Build history of the part. All positions in model axes, mm. Round coordinates to 2 decimals unless told otherwise and drop trailing zeros. Loops run counter-clockwise (first coordinate to the right, second up) from the corner with the lowest first, then second, coordinate; pieces in that order, holes last. Notation, with made-up numbers: (82.25, -1.5) -> (122.25, -1.5) arc R14 cw to (122.25, 19.5) -> close; hole circle Ø3 at (60, 11.25). An arc over 180 degrees is marked (long way). Put each result on its own line as item: value. Start each with the question number.
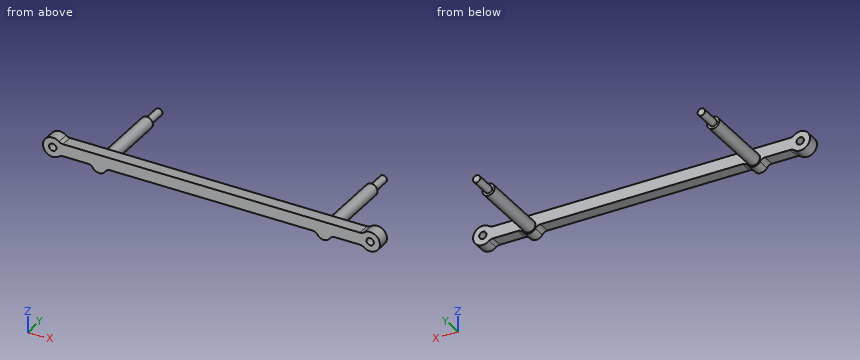
```python
from build123d import *

# Parameters (mm, degrees)
SKETCH1_R           = 1.5
BOSS_EXTRUDE1_DEPTH = 5
FILLET1_R           = 2.5
SKETCH2_R           = 2.5
BOSS_EXTRUDE2_DEPTH = 29
SKETCH3_R           = 1.5
BOSS_EXTRUDE3_DEPTH = 8.5


with BuildPart() as part:
    # Sketch1 → Boss-Extrude1 (new body)
    with BuildSketch(Plane(origin=(0, 0, 0), x_dir=(1, 0, 0), z_dir=(0, 1, 0))):
        with BuildLine():
            Line((-48.958039892, 2.5), (-61.877501001, 2.5))
            ThreePointArc((-61.877501001, 2.5), (-69, 0), (-61.877501001, -2.5))
            Line((-61.877501001, -2.5), (61.877501001, -2.5))
            ThreePointArc((61.877501001, -2.5), (69, 0), (61.877501001, 2.5))
            Line((61.877501001, 2.5), (48.958039892, 2.5))
            ThreePointArc((48.958039892, 2.5), (46, 5), (43.041960108, 2.5))
            Line((43.041960108, 2.5), (-43.041960108, 2.5))
            ThreePointArc((-43.041960108, 2.5), (-46, 5), (-48.958039892, 2.5))
        make_face()
        with Locations((-65, 0)):
            Circle(SKETCH1_R, mode=Mode.SUBTRACT)
        with Locations((65, 0)):
            Circle(SKETCH1_R, mode=Mode.SUBTRACT)
    extrude(amount=BOSS_EXTRUDE1_DEPTH)

    # Fillet1
    fillet1_edges = [part.edges().sort_by_distance(p)[0] for p in [
        (61.877501001, 2.5, -2.5),
        (61.877501001, 2.5, 2.5),
        (-61.877501001, 2.5, 2.5),
        (-61.877501001, 2.5, -2.5),
        (-48.958039892, 2.5, -2.5),
        (-43.041960108, 2.5, -2.5),
        (43.041960108, 2.5, -2.5),
        (48.958039892, 2.5, -2.5),
    ]]
    fillet(fillet1_edges, radius=FILLET1_R)

    # Sketch2 → Boss-Extrude2 (add)
    with BuildSketch(Plane(origin=(0, 5, 0), x_dir=(1, 0, 0), z_dir=(0, 1, 0))):
        with Locations((-46, 2)):
            Circle(SKETCH2_R)
        with Locations((46, 2)):
            Circle(SKETCH2_R)
    extrude(amount=BOSS_EXTRUDE2_DEPTH)

    # Sketch3 → Boss-Extrude3 (add)
    with BuildSketch(Plane(origin=(0, 34, 0), x_dir=(1, 0, 0), z_dir=(0, 1, 0))):
        with Locations((-46, 2)):
            Circle(SKETCH3_R)
        with Locations((46, 2)):
            Circle(SKETCH3_R)
    extrude(amount=BOSS_EXTRUDE3_DEPTH)


solid = part.part
```
Item 1: Cut at A-A on x = -65. Write the cut outline in (y, z), then the cut area to 3 significant figures.
Item 2: Cut at B-B on y = 13. Write the cut outline in (x, z).
Item 3: Cut at D-D on x = 37.5. Write the cut outline in (y, z), then the cut area to 3 significant figures.
Item 4: Drop flat-ended pins along their axis: pin 1 (5.5 mm diameter, centred on x = 14, y = 2.5, fed in from +Z); pin 2 (4 mm diameter, centred on x = -54, y = 2.5, fed in from -Z); pin 3 (4.5 mm diameter, centred on x = -10.5, z = -1.5, fed in from +Y). Give the stop position or say it passes through.
Item 5: Wall check: line 1 (X direction, y = 2.1, z = 0); line 2 (X direction, y = 9.5, z = -2); line 3 (Z direction, x = 65, y = 3). Give the ranges that are in metal, low to high. Write a range as from..to.
Item 6: Cut at C-C on x = -46. Write the cut outline in (y, z), then the cut area to 3 significant figures.
Ans:
1. outline: (0, -4) -> (5, -4) -> (5, -1.5) -> (0, -1.5) -> close; (0, 1.5) -> (5, 1.5) -> (5, 4) -> (0, 4) -> close
1. area: 25.0 mm2
2. outline: circle Ø5 at (-46, -2); circle Ø5 at (46, -2)
3. outline: (0, -2.5) -> (5, -2.5) -> (5, 2.5) -> (0, 2.5) -> close
3. area: 25.0 mm2
4. pin 1: stops at z = 2.5
4. pin 2: stops at z = -2.5
4. pin 3: stops at y = 5
5. line 1: x = -69..-66.5, -63.5..63.5, 66.5..69
5. line 2: x = -48.5..-43.5, 43.5..48.5
5. line 3: z = -4..-1.5, 1.5..4
6. outline: (0, -5) -> (5, -5) -> (5, -4.5) -> (34, -4.5) -> (34, -3.5) -> (42.5, -3.5) -> (42.5, -0.5) -> (34, -0.5) -> (34, 0.5) -> (5, 0.5) -> (5, 2.5) -> (0, 2.5) -> close
6. area: 208 mm2
